The listing builds one solid part. Answer for the finished solid, in the listing's coordinates (mm). Give positions to 0.01 mm unless a question says otherwise; leave off trailing zeros. Write each loop counter-clockwise with the first axis right and the second up, starting at its lowest first coordinate (ties: lowest second). Pieces come first, ordered by that corner, then holes. Notation, with made-up numbers: (13, 2) - (51, 2) arc R16 ccw to (51, 31) - close; hole circle Ø4 at (82, 70). An arc over 180 degrees is marked (long way). Answer as CSV lines item,"result". Start each with the question number.
(1) Find section A-A (x = 0). Write down the section's boundary in (y, z) (1 decimal).
(2) Find section C-C (x = 12). Write down the section's boundary in (y, z) (1 decimal).
(3) Straight lines are drawn through the part: probe 1 along Y at (x, z) = (0, -0.5); probe 2 along X at (y, z) = (-20, 2); probe 3 along X at (y, z) = (2, 0.25). For each, find the intervals that lie inside material, in ascending order.
(4) Find section B-B (y = 0). Write down the section's boundary in (x, z) (1 decimal).
(5) Each of these flat-tipped pins is pushed along its axis until it touches: pin 1 Ø1.5 at (y, z) = (-28, -2) entering from -X; pin 2 Ø3 at (x, z) = (-9.5, 2.5) entering from +Y; pin 3 Ø3 at (y, z) = (-22, -1) entering from -X; pin 4 Ø6.5 at (x, y) = (-11.91, 20.62) entering from +Z (3 decimals). Where does it stop, or does it pass through?
(6) For a pull along X with two mould halves and no side action, classify faces 1 (the face through (-11.012, -49.592, 0.044)), 2 (the face through (11, -11, -3.175)), 3 (the face through (10.03, -18.91, -0.04)) as pulls with the +X half, pulls with the -X half, needs draft (parallel to the pull), parting line crosses it, or undercut.
(7) Find section D-D (x = -24). Write down the section's boundary in (y, z) (3 decimals), then the cut area to 3 significant figures.
from build123d import *

# Parameters (mm, degrees)
F0_R     = 50.8
F0_R_2   = 2.54
F0_R_3   = 14.2875
F1_DEPTH = 3.175


with BuildPart() as f1:
    # F0 (on Top) → F1 (new body, symmetric)
    with BuildSketch(Plane.XY):
        Circle(F0_R)
        with Locations((-11.90625, -20.6222299276)):
            Circle(F0_R_2, mode=Mode.SUBTRACT)
        with Locations((-23.8125, 0)):
            Circle(F0_R_2, mode=Mode.SUBTRACT)
        Circle(F0_R_3, mode=Mode.SUBTRACT)
        with Locations((11.90625, -20.6222299276)):
            Circle(F0_R_2, mode=Mode.SUBTRACT)
        with Locations((23.8125, 0)):
            Circle(F0_R_2, mode=Mode.SUBTRACT)
        with Locations((-11.90625, 20.6222299276)):
            Circle(F0_R_2, mode=Mode.SUBTRACT)
        with Locations((11.90625, 20.6222299276)):
            Circle(F0_R_2, mode=Mode.SUBTRACT)
    extrude(amount=F1_DEPTH, both=True)


solid = f1.part
Result set:
1,outline,"(-50.8, -3.2) - (-14.3, -3.2) - (-14.3, 3.2) - (-50.8, 3.2) - close; (14.3, -3.2) - (50.8, -3.2) - (50.8, 3.2) - (14.3, 3.2) - close"
2,outline,"(-49.4, -3.2) - (-23.2, -3.2) - (-23.2, 3.2) - (-49.4, 3.2) - close; (-18.1, -3.2) - (-7.8, -3.2) - (-7.8, 3.2) - (-18.1, 3.2) - close; (7.8, -3.2) - (18.1, -3.2) - (18.1, 3.2) - (7.8, 3.2) - close; (23.2, -3.2) - (49.4, -3.2) - (49.4, 3.2) - (23.2, 3.2) - close"
3,probe 1,"-50.8 to -14.29, 14.29 to 50.8"
3,probe 2,"-46.7 to -14.37, -9.44 to 9.44, 14.37 to 46.7"
3,probe 3,"-50.76 to -25.38, -22.25 to -14.15, 14.15 to 22.25, 25.38 to 50.76"
4,outline,"(-50.8, -3.2) - (-26.4, -3.2) - (-26.4, 3.2) - (-50.8, 3.2) - close; (-21.3, -3.2) - (-14.3, -3.2) - (-14.3, 3.2) - (-21.3, 3.2) - close; (14.3, -3.2) - (21.3, -3.2) - (21.3, 3.2) - (14.3, 3.2) - close; (26.4, -3.2) - (50.8, -3.2) - (50.8, 3.2) - (26.4, 3.2) - close"
5,pin 1,"x = -42.87"
5,pin 2,"y = 50.17"
5,pin 3,"x = -46.48"
5,pin 4,"z = 3.175"
6,face 1,"parting line crosses it"
6,face 2,"needs draft"
6,face 3,"undercut"
7,outline,"(-44.773, -3.175) - (-2.533, -3.175) - (-2.533, 3.175) - (-44.773, 3.175) - close; (2.533, -3.175) - (44.773, -3.175) - (44.773, 3.175) - (2.533, 3.175) - close"
7,area,"536 mm^2"
